Geometry check sheet. Reference: the model listing, model coordinates, mm. Face numbers are marked on the shaded views. A direction names the side the tool comes from. Coordinates: 2 decimals unless noted, no trailing zeros. Loops run counter-clockwise (first coordinate to the right, second up) from the corner with the lowest first, then second, coordinate; pieces in that order, holes last.
from build123d import *

# Parameters (mm, degrees)
F2_R = 0.99999
F3_R = 5
F4_R = 10


# Not quite as in the source:
# - a fillet or chamfer is up to 0.001 mm smaller than in the source, because OpenCascade refuses the exact size


with BuildPart() as f1:
    # F0 (on Front) → F1 (revolve)
    with BuildSketch(Plane.XZ):
        Polygon((-11, 80), (-11, 0), (-9, 0), (-9, 80.6242772277), (-50.0682082509, 140), (-52.5, 140), align=None)
    revolve(axis=Axis((0, 0, 40), (0, 0, 1)))

    # F2 (radius 1 in the source; OpenCascade refuses exactly that, so slightly less here)
    f2_edges = [f1.edges().sort_by_distance(p)[0] for p in [
        (52.5, 0, 140),
        (50.068208, 0, 140),
        (11, 0, 0),
        (9, 0, 0),
    ]]
    fillet(f2_edges, radius=F2_R)

    # F3
    f3_edges = [f1.edges().sort_by_distance(p)[0] for p in [
        (9, 0, 80.624277),
    ]]
    fillet(f3_edges, radius=F3_R)

    # F4
    f4_edges = [f1.edges().sort_by_distance(p)[0] for p in [
        (11, 0, 80),
    ]]
    fillet(f4_edges, radius=F4_R)


solid = f1.part
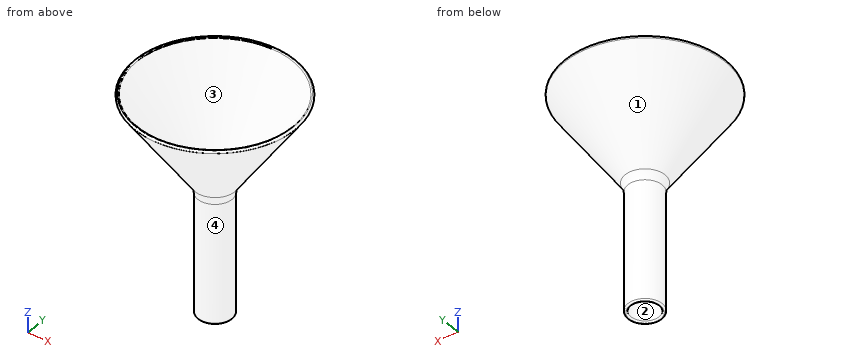
(1) Draft check along X on the marked faces 1 and 2. Enter one of: +X half, -X half, draft (parallel to the pull), parting line (faces both ways), or undercut.
Findings:
face 1: parting line
face 2: undercut
(2) Gauge pin test, flat ends, axial feed: pin 1 Ø10 at (x, z) = (-4.5, 42.5) entering from -Y; pin 2 Ø6 at (x, z) = (-22, 111) entering from -Y; pin 3 Ø8 at (y, z) = (-11.5, 36) entering from +X. Record the tip position at first contact, or that the pin passes through.
Findings:
pin 1: stops at y = -11
pin 2: stops at y = -27.48
pin 3: stops at x = 8.05
(3) Sectioned sample at B-B on z = 108.5. Record the cut outline in (x, y) (1 decimal).
Findings:
outline: circle Ø61.4 at (0, 0); hole circle Ø56.6 at (0, 0)
(4) Sectioned sample at A-A on z = 70. Record the cut outline in (x, y), and give its area (3 significant figures).
Findings:
outline: circle Ø22 at (0, 0); hole circle Ø18 at (0, 0)
area: 126 mm2
(5) Access from +Z, -Z, +X, -X, +Y, -Y to the whole of each face (thin tool, end or side, straight path). Record for the marked faces 3 and 4.
Findings:
face 3: +Z
face 4: -Z
(6) Scan lines: L1, parallel to Y at x = 0, z = 55; L2, parallel to X at y = 6.5, z = 8. Record each from-to range of solid material in increasing order.
Findings:
L1: y = -11 to -9, 9 to 11
L2: x = -8.87 to -6.22, 6.22 to 8.87
